Geometry: see drawing. Coordinates: mm, zero at the bounding-box minimum. A direction names the side the tool comes from. Coordinates: 2 decimals unless noted, no trailing zeros. Loops run counter-clockwise (first coordinate to the right, second up) from the corner with the lowest first, then second, coordinate; pieces in that order, holes last. Notation, with made-up numbers: (44.25, 64) - (95.25, 64) arc R18 ccw to (95.25, 75) - close; hole circle Ø5 at (5, 83.5). An arc over 180 degrees is marked (long way). Answer in a Markdown table with one row per item.
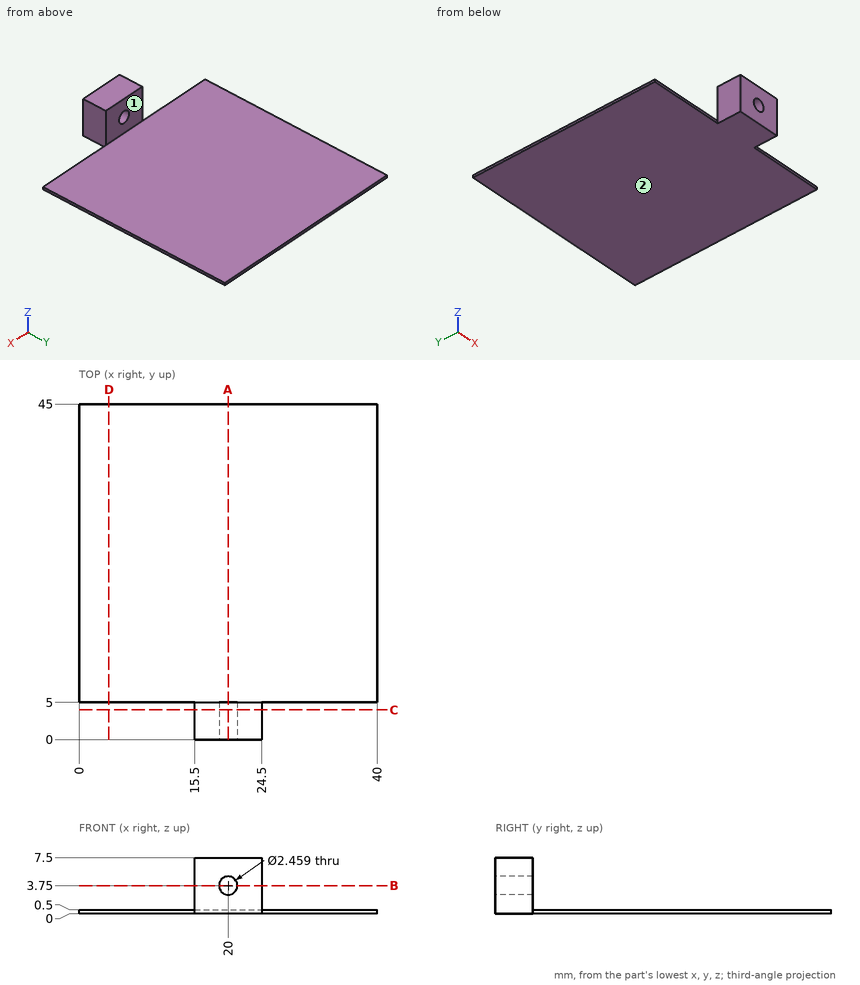
(1) Cut plane D-D on x = 4. Output: boundary loops of the cut face in (y, z).
Verdict:
| item | result |
|---|---|
| outline | (5, 0) - (45, 0) - (45, 0.5) - (5, 0.5) - close |
(2) Cut plane C-C on y = 4. Output: boundary loops of the cut face in (x, z).
Verdict:
| item | result |
|---|---|
| outline | (15.5, 0) - (24.5, 0) - (24.5, 7.5) - (15.5, 7.5) - close; hole circle Ø2.46 at (20, 3.75) |
(3) First-contact query: pin 1 Ø6 at (x, y) = (6.5, 9.5) entering from +Z; pin 2 Ø0.6 at (x, z) = (33, 0) entering from -Y; pin 3 Ø1.5 at (y, z) = (1.5, 5.5) entering from -X. Flat tips, straight axial feed; report the tip coordinate or a pass-through.
Verdict:
| item | result |
|---|---|
| pin 1 | stops at z = 0.5 |
| pin 2 | stops at y = 5 |
| pin 3 | stops at x = 15.5 |
(4) Access query for the marked faces 1 and 2. Directions: +Z, -Z, +X, -X, +Y, -Y. A direction counts if a zero-diameter tool reaches every point of the face in a straight line with its end or side. Return the directions, or none.
Verdict:
| item | result |
|---|---|
| face 1 | +Z, +X, -X, +Y |
| face 2 | -Z, +X, -X, +Y, -Y |
(5) Ray query, probe 1 along Z at (x, y) = (20, 2.6); probe 2 along X at (y, z) = (1.8, 3.75); probe 3 along Y at (x, z) = (16, 1.5). Return the intervals inside material, ascending.
Verdict:
| item | result |
|---|---|
| probe 1 | z = 0 to 2.52, 4.98 to 7.5 |
| probe 2 | x = 15.5 to 18.77, 21.23 to 24.5 |
| probe 3 | y = 0 to 5 |
(6) Cut plane A-A on x = 20. Output: boundary loops of the cut face in (y, z), then the cut area to 3 significant figures.
Verdict:
| item | result |
|---|---|
| outline | (0, 0) - (45, 0) - (45, 0.5) - (5, 0.5) - (5, 2.52) - (0, 2.52) - close; (0, 4.98) - (5, 4.98) - (5, 7.5) - (0, 7.5) - close |
| area | 45.2 mm² |
(7) Cut plane B-B on z = 3.75. Output: boundary loops of the cut face in (x, y).
Verdict:
| item | result |
|---|---|
| outline | (15.5, 0) - (18.77, 0) - (18.77, 5) - (15.5, 5) - close; (21.23, 0) - (24.5, 0) - (24.5, 5) - (21.23, 5) - close |
